from build123d import *

# Parameters (mm, degrees)
BOSS_EXTRUDE1_DEPTH      = 10
BOSS_EXTRUDE1_DEPTH_BACK = 23
SKETCH2_W                = 75
SKETCH2_H                = 18
CUT_EXTRUDE1_DEPTH       = 106.405673062
SKETCH3_W                = 4.26
SKETCH3_H                = 10
CUT_EXTRUDE2_DEPTH       = 103.075500294
CHAMFER1_SIZE            = 10
SKETCH4_R                = 2.75
CUT_EXTRUDE3_DEPTH       = 105.782669179
CUT_EXTRUDE4_DEPTH       = 90.13140726
CUT_EXTRUDE4_DEPTH_BACK  = 90.13140726
SKETCH5_R                = 3.25
SKETCH6_R                = 6
CUT_EXTRUDE5_DEPTH       = 96.528308685
CHAMFER2_SIZE            = 10
CHAMFER2_SIZE2           = 7.529686928
CUT_EXTRUDE6_DEPTH       = 102.066353255


with BuildPart() as part:
    # Sketch1 → Boss-Extrude1 (new, two sides: drawn at the far end of the back side and taken through both)
    with BuildSketch(Plane.XY.offset(-BOSS_EXTRUDE1_DEPTH_BACK)):
        Polygon((0, -7.5), (0, 7.5), (4.228226943, 7.5), (90, -32.313210233), (90, -42.313210233), (75, -42.313210233), align=None)
    extrude(amount=BOSS_EXTRUDE1_DEPTH + BOSS_EXTRUDE1_DEPTH_BACK)

    # Sketch2 → Cut-Extrude1 (cut, through all)
    with BuildSketch(Plane(origin=(0, 7.5, 0), x_dir=(1, 0, 0), z_dir=(0, 1, 0))):
        with Locations((52.5, 14)):
            Rectangle(SKETCH2_W, SKETCH2_H)
    extrude(amount=-CUT_EXTRUDE1_DEPTH, mode=Mode.SUBTRACT)

    # Sketch3 → Cut-Extrude2 (cut, through all)
    with BuildSketch(Plane(origin=(90, 0, 0), x_dir=(0, 0, -1), z_dir=(1, 0, 0))):
        with Locations((-1.63, -37.313210233)):
            Rectangle(SKETCH3_W, SKETCH3_H)
    extrude(amount=-CUT_EXTRUDE2_DEPTH, mode=Mode.SUBTRACT)

    # Chamfer1
    chamfer1_edges = [part.edges().sort_by_distance(p)[0] for p in [
        (15, -5.981321023, -5),
        (0, 0, 10),
    ]]
    chamfer(chamfer1_edges, length=CHAMFER1_SIZE)

    # Sketch4 → Cut-Extrude3 (cut, through all)
    with BuildSketch(Plane.XY.offset(10)):
        with Locations((80, -37.313210233)):
            Circle(SKETCH4_R)
    extrude(amount=-CUT_EXTRUDE3_DEPTH, mode=Mode.SUBTRACT)

    # Sketch5 → Cut-Extrude4 (cut, two sides: drawn at the far end of the back side and taken through both)
    with BuildSketch(Plane(origin=(15, 0, 0), x_dir=(0, 0, -1), z_dir=(1, 0, 0)).offset(-CUT_EXTRUDE4_DEPTH_BACK)):
        with Locations((15, -0.11657101)):
            Circle(SKETCH5_R)
    extrude(amount=CUT_EXTRUDE4_DEPTH + CUT_EXTRUDE4_DEPTH_BACK, mode=Mode.SUBTRACT)

    # Sketch6 → Cut-Extrude5 (cut, through all)
    with BuildSketch(Plane(origin=(7.5, 0, 0), x_dir=(0, 0, -1), z_dir=(1, 0, 0))):
        with Locations(Location((15, -0.11657101, 0), (0, 0, 181.598775169))):
            Circle(SKETCH6_R)
    extrude(amount=CUT_EXTRUDE5_DEPTH, mode=Mode.SUBTRACT)

    # Chamfer2
    chamfer2_edges = [part.edges().sort_by_distance(p)[0] for p in [
        (90, -32.313210233, 1.63),
    ]]
    chamfer2_side = [part.faces().sort_by_distance(p)[0] for p in [
        (43.268675536, -10.621644592, 0.683427775),
    ]]
    chamfer(chamfer2_edges, length=CHAMFER2_SIZE, length2=CHAMFER2_SIZE2, reference=chamfer2_side[0])

    # Sketch7 → Cut-Extrude6 (cut, through all)
    with BuildSketch(Plane(origin=(0, 0, -5), x_dir=(-1, 0, 0), z_dir=(0, 0, -1))):
        Polygon((-30, -19.12032651), (-70, -37.687371968), (-70, -37.787371968), (-30, -19.22032651), align=None)
        Polygon((-30, -17.12032651), (-70, -35.687371968), (-70, -35.787371968), (-30, -17.22032651), align=None)
        Polygon((-30, -15.12032651), (-70, -33.687371968), (-70, -33.787371968), (-30, -15.22032651), align=None)
        Polygon((-30, -13.12032651), (-70, -31.687371968), (-70, -31.787371968), (-30, -13.22032651), align=None)
        Polygon((-30, -11.12032651), (-70, -29.687371968), (-70, -29.787371968), (-30, -11.22032651), align=None)
        Polygon((-30, -9.12032651), (-70, -27.687371968), (-70, -27.787371968), (-30, -9.22032651), align=None)
        Polygon((-30, -7.12032651), (-70, -25.687371968), (-70, -25.787371968), (-30, -7.22032651), align=None)
    extrude(amount=-CUT_EXTRUDE6_DEPTH, mode=Mode.SUBTRACT)


solid = part.part
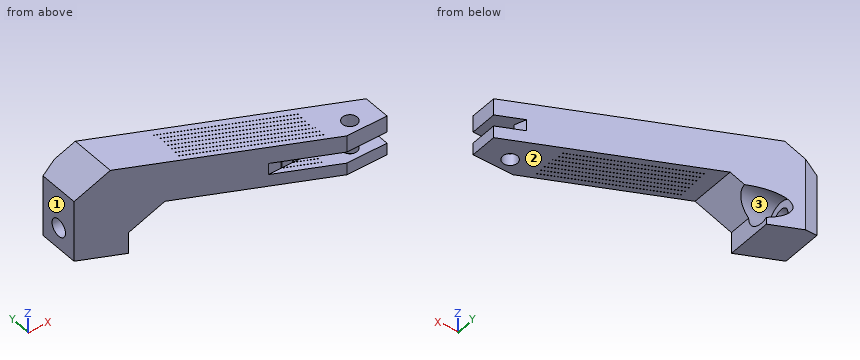
The listing builds one solid part. Answer for the finished solid, in the listing's coordinates (mm). Face numbers are marked on the shaded views. Round coordinates to 2 decimals unless told otherwise and drop trailing zeros. Order: outer loops, then holes, each group sorted by start corner. A loop starts at its lowest first (then second) coordinate and runs counter-clockwise, first axis right, second up. Notation, with made-up numbers: M 65.25,87 L 72.25,87 A15 ccw 72.25,115 Z; hole C 15,40 d4. An arc over 180 degrees is marked long. Answer in a Markdown table with one row per item. Add a question column.
1) Consider line 1 along Y through (x, z) = (80, 8.5); line 2 along X through (y, z) = (-30.5, -3); line 3 along X through (y, z) = (-36, 5). Determine where each line is inside the solid, lowest interval first. Write a range as from..to.
2) The part is cut by section D-D on z = -10. Determine the outline of the cut face in (x, y).
3) The part is cut by section A-A on x = 41.5. Count the separate pieces of the cut face and the enclosed holes in it, plus the area to 3 significant figures.
4) Flat-ended cylindrical pins translate along their axes: pin 1 Ø8 at (x, z) = (63, -4) entering from +Y; pin 2 Ø13 at (y, z) = (-1.5, -14.5) entering from +X; pin 3 Ø4 at (x, z) = (19, -1) entering from +Y. Find the tip coordinate at first contact, or state that the pin passes through.
5) The part is cut by section B-B on x = 80. Determine the outline of the cut face in (y, z), plus the area to 3 significant figures.
6) Determine the mould class of the marked faces 1, 2 and 3 for opening direction Z: pulls with the +Z half, pulls with the -Z half, needs draft (parallel to the pull), parting line crosses it, or undercut.
7) The part is cut by section C-C on z = -17. Determine the outline of the cut face in (x, y), plus the area to 3 significant figures.
Findings below:
| question | item | result |
|---|---|---|
| 1 | line 1 | y = -42.31..-40.06, -34.56..-27.67 |
| 1 | line 2 | x = 49.55..54.3, 54.52..58.61, 58.82..62.92, 63.13..67.23, 67.44..86.09 |
| 1 | line 3 | x = 61.4..66.15, 66.36..77.58, 82.42..90 |
| 2 | outline | M 0,-7.5 L 20,-16.78 L 20,-3.43 L 7.5,-3.43 L 7.5,3.2 L 13.49,3.2 L 4.23,7.5 L 0,7.5 Z |
| 3 | separate pieces | 8 |
| 3 | enclosed holes | 0 |
| 3 | area | 244 mm² |
| 4 | pin 1 | stops at y = -17.92 |
| 4 | pin 2 | stops at x = 22 |
| 4 | pin 3 | stops at y = 1.57 |
| 5 | outline | M -42.31,-5 L -40.06,-5 L -40.06,-0.5 L -42.31,-0.5 Z; M -42.31,3.76 L -40.06,3.76 L -40.06,10 L -42.31,10 Z; M -34.56,-5 L -27.67,-5 L -27.67,10 L -34.56,10 L -34.56,3.76 L -32.31,3.76 L -32.31,-0.5 L -34.56,-0.5 Z |
| 5 | area | 118 mm² |
| 6 | face 1 | needs draft |
| 6 | face 2 | pulls with the -Z half |
| 6 | face 3 | undercut |
| 7 | outline | M 0,-7.5 L 15,-14.46 L 15,-5.77 L 7.5,-5.77 L 7.5,-2.68 L 0,-2.68 Z; M 0,2.45 L 7.5,2.45 L 7.5,5.54 L 8.45,5.54 L 4.23,7.5 L 0,7.5 Z |
| 7 | area | 137 mm² |
